Geometry: see drawing. Coordinates: mm, zero at the bounding-box minimum. A direction names the side the tool comes from. Give positions to 0.01 mm unless a question says otherwise; leave off trailing zeros. Write each loop counter-clockwise with the first axis right and the second up, starting at its lowest first coordinate (ties: lowest second). Pieces come first, ordered by that corner, then holes. Notation, with made-up numbers: M -1.75,49.25 L 26.25,49.25 A20 ccw 26.25,66.25 Z; hole C 64.25,87 d3. An arc over 180 degrees is marked long. Use CSV: the item, a comma, the result in double quotes. Start each with the question number.
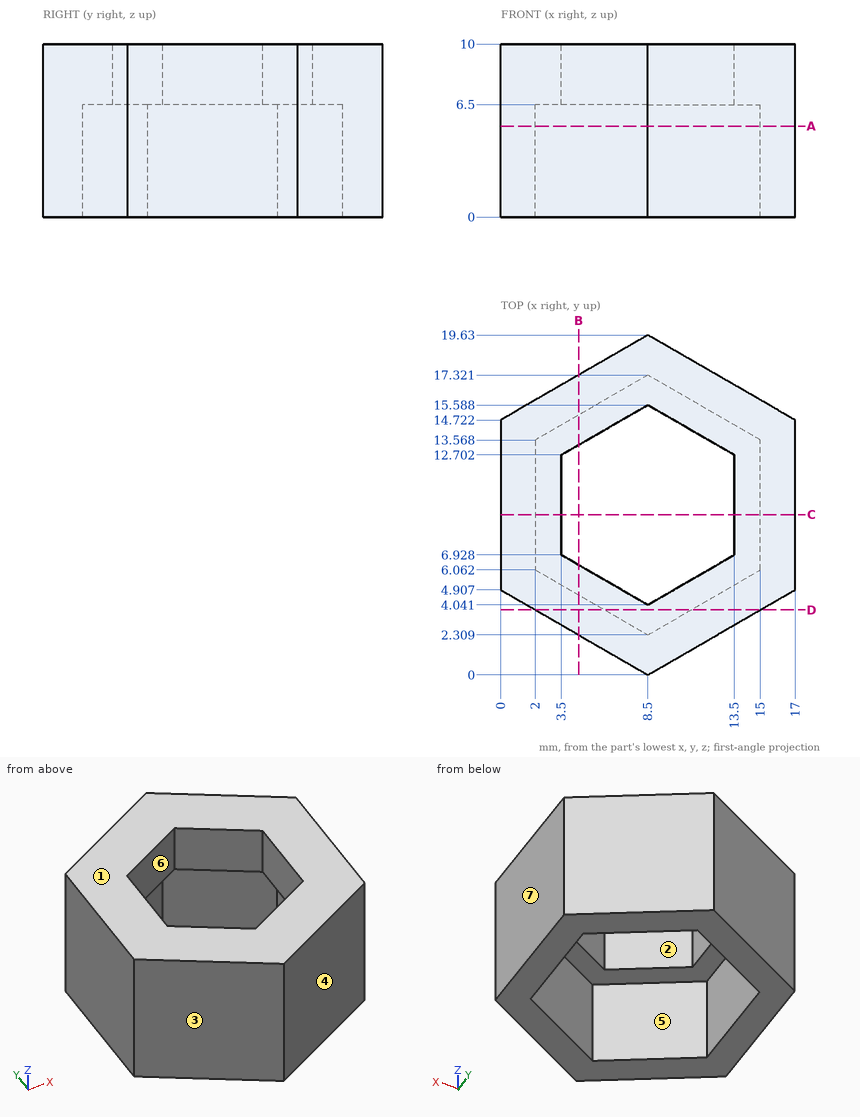
1. Section B-B on x = 4.5. Return loops of the section in (y, z).
2. Pull-direction query (X, two-part tool) for the marked faces 1, 2, 3 and 4; classes: released by +X, released by -X, zero draft, split by the parting line, or undercut.
3. First-contact query: pin 1 (2 mm diameter, centred on x = 10, y = 5, fed in from -Z); pin 2 (1 mm diameter, centred on x = 14, z = 2, fed in from +Y); pin 3 (2 mm diameter, centred on x = 14, z = 4.5, fed in from +Y). Flat tips, straight axial feed; report the tip coordinate or a pass-through.
4. Section A-A on z = 5.25. Return loops of the section in (x, y), then the cut area to 3 significant figures.
5. Access query for the marked faces 5, 6 and 7. Directions: +Z, -Z, +X, -X, +Y, -Y. A direction counts if a zero-diameter tool reaches every point of the face in a straight line with its end or side. Return the directions, or none.
6. Line query: probe 1 along X at (y, z) = (10.25, 9); probe 2 along X at (y, z) = (7.25, 2.25); probe 3 along Z at (x, y) = (14.25, 9.75). Output: solid intervals per line, ascending.
7. Section D-D on y = 3.75. Return loops of the section in (x, z) (1 decimal).
8. Section C-C on y = 9.25. Return loops of the section in (x, z).
Resolved:
1,outline,"M 2.31,0 L 4.62,0 L 4.62,6.5 L 6.35,6.5 L 6.35,10 L 2.31,10 Z; M 13.28,6.5 L 15.01,6.5 L 15.01,0 L 17.32,0 L 17.32,10 L 13.28,10 Z"
2,face 1,"zero draft"
2,face 2,"undercut"
2,face 3,"released by -X"
2,face 4,"released by +X"
3,pin 1,"stops at z = 6.5"
3,pin 2,"stops at y = 16.74"
3,pin 3,"stops at y = 17.03"
4,outline,"M 0,4.91 L 8.5,0 L 17,4.91 L 17,14.72 L 8.5,19.63 L 0,14.72 Z; hole M 2,6.06 L 8.5,2.31 L 15,6.06 L 15,13.57 L 8.5,17.32 L 2,13.57 Z"
4,area,"104 mm2"
5,face 5,"-Z"
5,face 6,"+Z, -Z"
5,face 7,"+Z, -Z, +X, +Y, -Y"
6,probe 1,"x = 0 to 3.5, 13.5 to 17"
6,probe 2,"x = 0 to 2, 15 to 17"
6,probe 3,"z = 6.5 to 10"
7,outline,"M 2,0 L 6,0 L 6,6.5 L 11,6.5 L 11,0 L 15,0 L 15,10 L 2,10 Z"
8,outline,"M 0,0 L 2,0 L 2,6.5 L 3.5,6.5 L 3.5,10 L 0,10 Z; M 13.5,6.5 L 15,6.5 L 15,0 L 17,0 L 17,10 L 13.5,10 Z"
